Geometry check sheet. Reference: the model listing, model coordinates, mm. A direction names the side the tool comes from. Give positions to 0.01 mm unless a question says otherwise; leave off trailing zeros. Write each loop counter-clockwise with the first axis right and the second up, starting at its lowest first coordinate (ties: lowest second). Pieces come first, ordered by that corner, then holes.
(1) Cross-section at A-A (z = 1.5). Record the boundary of the cut face in (x, y), and give its area (3 significant figures).
(2) Thickness scan on line 1 along Y through (x, z) = (31.5, -6); line 2 along Z through (x, y) = (27.5, -94.65); line 3 along Z through (x, y) = (4.4, 0.8). Record the ranges inside material, lowest first.
(3) Tool access check on faces 1 (the flat face through (6, -46, 3)), 2 (the flat face through (49, -47, 3)), 3 (the flat face through (13.9, -95.37, -12.01)). Record the directions out of +Z, -Z, +X, -X, +Y, -Y that give a thin tool (end or side, any length) a straight path to the whole face; none if there is none.
(4) Cross-section at C-C (y = -8). Record the boundary of the cut face in (x, z).
(5) Mould release check, pull along Z, two halves, no side actions. Record for faces 4 (the flat face through (15.902, 1.972, -17.713)), 5 (the cylindrical face through (28.58, -95.07, -18.82)), 6 (the cylindrical face through (51.081, 1.065, -17.974)), 7 (the flat face through (51.958, -17.487, 2.958)): +Z half, -Z half, draft (parallel to the pull), parting line (faces both ways), or undercut.
(6) Depth check by flat-ended pin: P1, Ø3, axis at x = 26.5, y = 2.5, coming from the -Z side; P2, Ø3, axis at x = 25.5, y = -95, coming from the -Z side; P3, Ø5, axis at y = -35, z = 2, coming from the +X side; P4, Ø12, axis at x = 37, z = -21, coming from the +Y side. Enter the tip coordinate at first touch or a pass-through.
(7) Cross-section at D-D (z = -19.5). Count the separate pieces of the cut face and the enclosed holes in it, and give its area (3 significant figures).
(8) Cross-section at B-B (x = 36). Record the boundary of the cut face in (y, z), and give its area (3 significant figures).
```python
from build123d import *

# Parameters (mm, degrees)
BOSS_EXTRUDE1_DEPTH = 6
BOSS_EXTRUDE2_DEPTH = 4
BOSS_EXTRUDE3_DEPTH = 4
SKETCH4_R           = 2.7
CUT_EXTRUDE1_DEPTH  = 6
SKETCH6_R           = 5.6
SKETCH5_R           = 2.7
SKETCH7_R           = 1.6
CUT_EXTRUDE2_DEPTH  = 4
SKETCH8_R           = 1.6
CUT_EXTRUDE3_DEPTH  = 4
LPATTERN1_COUNT     = 2
LPATTERN1_PITCH     = 46.2


with BuildPart() as part:
    # Sketch1 → Boss-Extrude1 (new body)
    with BuildSketch(Plane.XY):
        Polygon((55, 0), (0, 0), (0, -13.787434686), (6, -21.083714938), (6, -72.316285062), (0, -79.612565314), (0, -93.4), (55, -93.4), (55, -79.612565314), (49, -72.316285062), (49, -21.083714938), (55, -13.787434686), align=None)
    extrude(amount=BOSS_EXTRUDE1_DEPTH)

    # Sketch2 → Boss-Extrude2 (add)
    with BuildSketch(Plane(origin=(0, 0, 0), x_dir=(1, 0, 0), z_dir=(0, 1, 0))):
        Polygon((0, -6), (0, 0), (0, 24.368247755), (10.336028335, 24.368247755), (21.625062203, 10.869324577), (33.374937797, 10.869324577), (44.663971665, 24.368247755), (55, 24.368247755), (55, 0), (55, -6), align=None)
    extrude(amount=BOSS_EXTRUDE2_DEPTH)

    # Sketch3 → Boss-Extrude3 (add)
    with BuildSketch(Plane.XZ.offset(93.4)):
        Polygon((55, 6), (0, 6), (0, 0), (7.974588669, 0), (20, -24.364916427), (35, -24.364916427), (47.025411331, 0), (55, 0), align=None)
    extrude(amount=BOSS_EXTRUDE3_DEPTH)

    # Sketch4 → Cut-Extrude1 (cut)
    with BuildSketch(Plane.XY.offset(6)):
        with Locations((27.5, -48.6)):
            Circle(SKETCH4_R)
    extrude(amount=-CUT_EXTRUDE1_DEPTH, mode=Mode.SUBTRACT)

    # Sketch6 → Cut-Loft1 section 0
    with BuildSketch(Plane.XY.offset(6)):
        with Locations((27.5, -48.6)):
            Circle(SKETCH6_R)
    # Sketch5 → Cut-Loft1 section 1
    with BuildSketch(Plane.XY.offset(2.85)):
        with Locations((27.5, -48.6)):
            Circle(SKETCH5_R)
    loft(mode=Mode.SUBTRACT)

    # Sketch7 → Cut-Extrude2 (cut)
    with BuildSketch(Plane(origin=(0, 4, 0), x_dir=(1, 0, 0), z_dir=(0, 1, 0))):
        with Locations(Location((50.6, 19.5, 0), (0, 0, 270))):
            Circle(SKETCH7_R)
        with Locations(Location((4.4, 19.5, 0), (0, 0, 270))):
            Circle(SKETCH7_R)
    extrude(amount=-CUT_EXTRUDE2_DEPTH, mode=Mode.SUBTRACT)

    # Sketch8 → Cut-Extrude3 (cut)
    with BuildSketch(Plane.XZ.offset(97.4)):
        with Locations(Location((27.5, -20, 0), (0, 0, 270))):
            Circle(SKETCH8_R)
    extrude(amount=-CUT_EXTRUDE3_DEPTH, mode=Mode.SUBTRACT)

    # Cut-Loft2: read off the stored shape, not the designer's step
    # Cut-Loft2: loft between two sections, ruled curve by curve
    cut_loft2_from = [
        Edge.make_bspline([(28.144905496, -97.4, -16.687188218), (34.77052906, -97.4, -17.97699921), (33.480718067, -97.4, -24.602622774), (26.855094504, -97.4, -23.312811782), (20.22947094, -97.4, -22.02300079), (21.519281933, -97.4, -15.397377226), (28.144905496, -97.4, -16.687188218)], [0, 0, 0, 0, 0.5, 0.5, 0.5, 1, 1, 1, 1], 3, [1, 0.333333333, 0.333333333, 1, 0.333333333, 0.333333333, 1]),
    ]
    cut_loft2_to = [
        Edge.make_bspline([(26.657155547, -95.5, -21.360004864), (23.93714582, -95.5, -19.674315958), (25.622834725, -95.5, -16.954306231), (28.342844453, -95.5, -18.639995136), (31.06285418, -95.5, -20.325684042), (29.377165275, -95.5, -23.045693769), (26.657155547, -95.5, -21.360004864)], [0, 0, 0, 0, 0.5, 0.5, 0.5, 1, 1, 1, 1], 3, [1, 0.333333333, 0.333333333, 1, 0.333333333, 0.333333333, 1]),
    ]
    cut_loft2 = Solid(Shell([*[Face.make_surface_from_curves(cut_loft2_from[k], cut_loft2_to[k]) for k in range(1)], Face(Wire(cut_loft2_from)), Face(Wire(cut_loft2_to))]))
    add(cut_loft2, mode=Mode.SUBTRACT)

    # Cut-Loft3: read off the stored shape, not the designer's step
    # Cut-Loft3: loft between two sections, ruled curve by curve
    cut_loft3_from = [
        Edge.make_bspline([(50.313932129, 4, -22.862854468), (57.039641066, 4, -23.434990209), (57.611776807, 4, -16.709281273), (50.886067871, 4, -16.137145532), (44.160358934, 4, -15.565009791), (43.588223193, 4, -22.290718727), (50.313932129, 4, -22.862854468)], [0, 0, 0, 0, 0.5, 0.5, 0.5, 1, 1, 1, 1], 3, [1, 0.333333333, 0.333333333, 1, 0.333333333, 0.333333333, 1]),
    ]
    cut_loft3_to = [
        Edge.make_bspline([(50.101749949, 2.1, -21.02044299), (53.14263593, 2.1, -22.016943092), (54.139136031, 2.1, -18.976057111), (51.098250051, 2.1, -17.97955701), (48.05736407, 2.1, -16.983056908), (47.060863969, 2.1, -20.023942889), (50.101749949, 2.1, -21.02044299)], [0, 0, 0, 0, 0.5, 0.5, 0.5, 1, 1, 1, 1], 3, [1, 0.333333333, 0.333333333, 1, 0.333333333, 0.333333333, 1]),
    ]
    cut_loft3 = Solid(Shell([*[Face.make_surface_from_curves(cut_loft3_from[k], cut_loft3_to[k]) for k in range(1)], Face(Wire(cut_loft3_from)), Face(Wire(cut_loft3_to))]))
    add(cut_loft3, mode=Mode.SUBTRACT)

    # LPattern1: Cut-Loft3 ×2
    with Locations(*[(-i * LPATTERN1_PITCH, 0, 0) for i in range(1, LPATTERN1_COUNT)]):
        add(cut_loft3, mode=Mode.SUBTRACT)


solid = part.part
```
Reply:
1. outline: (0, -97.4) - (55, -97.4) - (55, -79.61) - (49, -72.32) - (49, -21.08) - (55, -13.79) - (55, 4) - (0, 4) - (0, -13.79) - (6, -21.08) - (6, -72.32) - (0, -79.61) - close; hole circle Ø5.4 at (27.5, -48.6)
1. area: 4,850 mm2
2. line 1: y = -97.4 to -93.4, 0 to 4
2. line 2: z = -24.36 to -21.6, -18.4 to 6
2. line 3: z = -24.37 to -21.1, -17.9 to 6
3. face 1: +Z, -Z, -X
3. face 2: +Z, -Z, +X
3. face 3: -Z, -X, -Y
4. outline: (0, 0) - (55, 0) - (55, 6) - (0, 6) - close
5. face 4: -Z half
5. face 5: undercut
5. face 6: undercut
5. face 7: draft
6. P1: stops at z = -10.87
6. P2: stops at z = -24.36
6. P3: stops at x = 49
6. P4: stops at y = 4
7. separate pieces: 6
7. enclosed holes: 0
7. area: 149 mm2
8. outline: (-97.4, -22.34) - (-93.4, -22.34) - (-93.4, 0) - (0, 0) - (0, -14.01) - (4, -14.01) - (4, 6) - (-97.4, 6) - close
8. area: 754 mm2
